from build123d import *

# Parameters (mm, degrees)
F0_W        = 95.25
F0_H        = 25.4
F1_DEPTH    = 12.7
F2_W        = 127
F2_H        = 76.2
F3_DEPTH    = 2.54
F4_T        = 2.54
F4_T3_DEPTH = 100.33
F4_T5_DEPTH = 30.48
F5_DEPTH    = 25.4
F6_DEPTH    = 25.4
F7_DEPTH    = 25.4
F10_DEPTH   = 5.08


# Not quite as in the source:
# - a shell that OpenCascade refuses in one call is made with other operations: the cavity is built on its own and cut out


with BuildPart() as f1:
    # F0 (on Top) → F1 (new body)
    with BuildSketch(Plane.XY):
        Rectangle(F0_W, F0_H)
    extrude(amount=F1_DEPTH)

    # F2 (on Top) → F3 (join)
    with BuildSketch(Plane.XY):
        Rectangle(F2_W, F2_H)
    extrude(amount=-F3_DEPTH)

    # F4: shell of thickness 2.54, made by hand


with BuildPart() as f4_core1:
    # F4_t2: copy of F1
    add(f1.part)

    # the walls: a layer under each face that stays
    f4_faces = [f4_core1.faces().sort_by_distance(p)[0] for p in [
        (63.5, 0, -1.27),
        (0, -38.1, -1.27),
        (0, 38.1, -1.27),
        (-42.3333333333, -25.4, 0),
        (0, 0, -2.54),
        (-63.5, 0, -1.27),
        (0, -12.7, 6.35),
        (47.625, 0, 6.35),
        (0, 12.7, 6.35),
        (-47.625, 0, 6.35),
    ]]
    thicken(f4_faces, amount=-F4_T, mode=Mode.SUBTRACT)

    # F4_s4 → F4_t3 (cut)
    with BuildSketch(Plane.YZ.offset(-50.165)):
        Polygon((-12.7254, 0.0254), (-12.7, -2.54), (-10.16, -2.54), (-10.16, 0), align=None)
        Polygon((12.7254, 0.0254), (12.7, -2.54), (10.16, -2.54), (10.16, 0), align=None)
    extrude(amount=F4_T3_DEPTH, mode=Mode.SUBTRACT)

    # F4_s6 → F4_t5 (cut)
    with BuildSketch(Plane.XZ.offset(-15.24)):
        Polygon((47.6504, 0.0254), (47.625, -2.54), (45.085, -2.54), (45.085, 0), align=None)
        Polygon((-47.6504, 0.0254), (-47.625, -2.54), (-45.085, -2.54), (-45.085, 0), align=None)
    extrude(amount=F4_T5_DEPTH, mode=Mode.SUBTRACT)


with BuildPart() as f1_1:
    add(f1.part)

    # what is left inside the walls is the cavity
    f4_cavity = [f4_core1.part.solids().sort_by_distance(p)[0] for p in [
        (0, -3.386667, 0.0254),
    ]]
    add(f4_cavity, mode=Mode.SUBTRACT)

    # F5 (cut): a face of the model
    f5_faces = [f1_1.faces().sort_by_distance(p)[0] for p in [
        (-45.085, 0, 6.35),
    ]]
    extrude(f5_faces, amount=-F5_DEPTH, mode=Mode.SUBTRACT)

    # F6 (cut): a face of the model
    f6_faces = [f1_1.faces().sort_by_distance(p)[0] for p in [
        (45.085, 0, 6.35),
    ]]
    extrude(f6_faces, amount=-F6_DEPTH, mode=Mode.SUBTRACT)

    # F7 (add): a face of the model
    f7_faces = [f1_1.faces().sort_by_distance(p)[0] for p in [
        (0, 11.43, 12.7),
    ]]
    extrude(f7_faces, amount=F7_DEPTH)

    # F9 (on face) → F10 (cut)
    with BuildSketch(Plane.XZ.offset(12.7)):
        with BuildLine():
            ThreePointArc((7.7229928646, 12.7), (7.7554155926, 13.1086234281), (7.7662332139, 13.5183883831))
            ThreePointArc((7.7662332139, 13.5183883831), (-0.409764955, 21.2738039757), (-7.7229928646, 12.7))
            Line((-7.7229928646, 12.7), (7.7229928646, 12.7))
        make_face()
        with BuildLine():
            Line((7.7229928646, 12.7), (-7.7229928646, 12.7))
            ThreePointArc((-7.7229928646, 12.7), (0, 5.7521551692), (7.7229928646, 12.7))
        make_face()
    extrude(amount=-F10_DEPTH, mode=Mode.SUBTRACT)


solid = f1_1.part
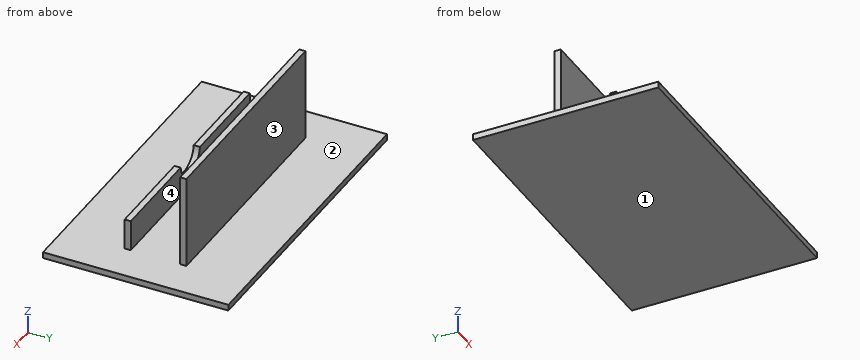
Input: part model. Units: mm. Frame: model coordinates. Face numbers are marked on the shaded views. Coordinates: 2 decimals unless noted, no trailing zeros. Loops run counter-clockwise (first coordinate to the right, second up) from the corner with the lowest first, then second, coordinate; pieces in that order, holes last. Notation, with made-up numbers: (56, -20.5) -> (113, -20.5) arc R16 ccw to (113, 6.5) -> close; hole circle Ø2 at (12, 41). An arc over 180 degrees is marked (long way). Write item = value, one per line. Start each with the question number.
Item 1: Cut plane C-C, the plane y = -18. Return loops of the section in (x, z).
Item 2: First-contact query: P1, Ø12, axis at x = 2.5, z = 8.5, coming from the -Y side; P2, Ø0.8, axis at y = -12, z = 7.5, coming from the +X side (3 decimals); P3, Ø1.3, axis at x = 32.5, y = -11.5, coming from the +Z side; P4, Ø14, axis at x = -4.5, z = 6, coming from the +Y side. Flat tips, straight axial feed; report the tip coordinate or a pass-through.
Item 3: Cut plane A-A, the plane x = 30. Return loops of the section in (y, z).
Item 4: Cut plane B-B, the plane z = 30. Return loops of the section in (x, y) (3 decimals), plus the area to 3 significant figures.
Item 5: Mould query, pull axis Y, two halves, no side actions, for the marked faces 1, 2, 3 and 4. Classes: pulls with the +Y half, pulls with the -Y half, needs draft (parallel to the pull), parting line crosses it, or undercut.
Item 6: Material intervals for line 1 (Y direction, x = 4, z = 1); line 2 (Z direction, x = -47.5, y = -6.5); line 3 (Y direction, x = -26, z = 27.5), sorted ascending.
Ans:
q1.outline = (-63.5, -2.54) -> (63.5, -2.54) -> (63.5, 0) -> (-63.5, 0) -> close
q2.P1 = -12.7
q2.P2 = 47.625
q2.P3 = 12.7
q2.P4 = 38.1
q3.outline = (-38.1, -2.54) -> (38.1, -2.54) -> (38.1, 0) -> (12.7, 0) -> (12.7, 38.1) -> (10.16, 38.1) -> (10.16, 0) -> (-10.16, 0) -> (-10.16, 12.7) -> (-12.7, 12.7) -> (-12.7, 0) -> (-38.1, 0) -> close
q4.outline = (-47.625, 10.16) -> (47.625, 10.16) -> (47.625, 12.7) -> (-47.625, 12.7) -> close
q4.area = 242 mm²
q5.face_1 = needs draft
q5.face_2 = undercut
q5.face_3 = pulls with the +Y half
q5.face_4 = undercut
q6.line_1 = -12.7 to -10.16, 10.16 to 12.7
q6.line_2 = -2.54 to 0
q6.line_3 = 10.16 to 12.7
